```python
from build123d import *

# Parameters (mm, degrees)
SKETCH_W     = 52
SKETCH_H     = 52
SKETCH_R     = 1.8
SKETCH_R_2   = 1.5
SKETCH_W_2   = 38
SKETCH_H_2   = 7.5
PAD_DEPTH    = 2
SKETCH001_W  = 25.7
SKETCH001_H  = 8
POCKET_DEPTH = 5


with BuildPart() as part:
    # Sketch → Pad (new body)
    with BuildSketch(Plane.XY):
        Rectangle(SKETCH_W, SKETCH_H)
        with Locations((22.25, 22.25)):
            Circle(SKETCH_R, mode=Mode.SUBTRACT)
        with Locations((22.25, -22.25)):
            Circle(SKETCH_R, mode=Mode.SUBTRACT)
        with Locations((-22.25, 22.25)):
            Circle(SKETCH_R, mode=Mode.SUBTRACT)
        with Locations((-22.25, -22.25)):
            Circle(SKETCH_R, mode=Mode.SUBTRACT)
        with Locations((16.25, 8.55)):
            Circle(SKETCH_R_2, mode=Mode.SUBTRACT)
        with Locations((-16.25, 8.76716)):
            Circle(SKETCH_R_2, mode=Mode.SUBTRACT)
        with Locations((-16.25, -8.53284)):
            Circle(SKETCH_R_2, mode=Mode.SUBTRACT)
        with Locations((16.25, -8.75)):
            Circle(SKETCH_R_2, mode=Mode.SUBTRACT)
        with Locations((0, 15.25)):
            Rectangle(SKETCH_W_2, SKETCH_H_2, mode=Mode.SUBTRACT)
        with Locations((0, -15.25)):
            Rectangle(SKETCH_W_2, SKETCH_H_2, mode=Mode.SUBTRACT)
    extrude(amount=PAD_DEPTH)

    # Sketch001 → Pocket (cut)
    with BuildSketch(Plane.XY.offset(2)):
        with Locations((0, -10.5)):
            Rectangle(SKETCH001_W, SKETCH001_H)
    extrude(amount=-POCKET_DEPTH, mode=Mode.SUBTRACT)


solid = part.part
```
Geometry check sheet. Reference: the model listing, model coordinates, mm. A direction names the side the tool comes from. Give positions to 0.01 mm unless a question says otherwise; leave off trailing zeros. Write each loop counter-clockwise with the first axis right and the second up, starting at its lowest first coordinate (ties: lowest second). Pieces come first, ordered by that corner, then holes.
1) Section check A-A, the plane x = 2.5. Record the boundary of the cut face in (y, z).
2) Material ranges on L1, parallel to Y at x = 4, z = 0.75; L2, parallel to Y at x = -22.25, z = 0.75; L3, parallel to X at y = 12, z = 0.6, recorded low to high.
3) Release check for a two-part mould opening along Y. For faces 3 (the flat face through (0, -26, 1)), 4 (the flat face through (0, 0, 0)), 5 (the flat face through (19, 15, 1)) record: pulls with the +Y half, pulls with the -Y half, needs draft (parallel to the pull), parting line crosses it, or undercut.
4) Gauge pin test, flat end, axial feed: pin 1 (2.5 mm diameter, centred on x = 16.25, y = 8.55, fed in from -Z). Record the tip position at first contact, or that the pin passes through.
5) Section check B-B, the plane y = -22.25. Record the boundary of the cut face in (x, z), and give its area (3 significant figures).
6) Section check D-D, the plane y = 13. Record the boundary of the cut face in (x, z).
7) Section check C-C, the plane x = -16.25. Record the boundary of the cut face in (y, z).
8) Access from +Z, -Z, +X, -X, +Y, -Y to the whole of each face (thin tool, end or side, straight path). Record for faces 1 (the flat face through (-26, 0, 1)), 2 (the flat face through (0, -6.5, 1)).
Computed:
1. outline: (-26, 0) - (-19, 0) - (-19, 2) - (-26, 2) - close; (-6.5, 0) - (11.5, 0) - (11.5, 2) - (-6.5, 2) - close; (19, 0) - (26, 0) - (26, 2) - (19, 2) - close
2. L1: y = -26 to -19, -6.5 to 11.5, 19 to 26
2. L2: y = -26 to -24.05, -20.45 to 20.45, 24.05 to 26
2. L3: x = -26 to -19, 19 to 26
3. face 3: pulls with the -Y half
3. face 4: needs draft
3. face 5: undercut
4. pin 1: passes through
5. outline: (-26, 0) - (-24.05, 0) - (-24.05, 2) - (-26, 2) - close; (-20.45, 0) - (20.45, 0) - (20.45, 2) - (-20.45, 2) - close; (24.05, 0) - (26, 0) - (26, 2) - (24.05, 2) - close
5. area: 89.6 mm2
6. outline: (-26, 0) - (-19, 0) - (-19, 2) - (-26, 2) - close; (19, 0) - (26, 0) - (26, 2) - (19, 2) - close
7. outline: (-26, 0) - (-19, 0) - (-19, 2) - (-26, 2) - close; (-11.5, 0) - (-10.03, 0) - (-10.03, 2) - (-11.5, 2) - close; (-7.03, 0) - (7.27, 0) - (7.27, 2) - (-7.03, 2) - close; (10.27, 0) - (11.5, 0) - (11.5, 2) - (10.27, 2) - close; (19, 0) - (26, 0) - (26, 2) - (19, 2) - close
8. face 1: +Z, -Z, -X, +Y, -Y
8. face 2: +Z, -Z
